from build123d import *
from build123d.topology import SkipClean

# Parameters (mm, degrees)
BOSS_EXTRUDE1_DEPTH  = 20
SKETCH2_W            = 53
SKETCH2_H            = 20
CUT_EXTRUDE1_DEPTH   = 20
FILLET1_R            = 9.75
FILLET1_OF_MIRROR4_R = 9.75
SKETCH4_R            = 2.1
CUT_EXTRUDE3_DEPTH   = 20
FILLET2_R            = 20


with BuildPart() as part:
    # Sketch1 → Boss-Extrude1 (new body)
    with BuildSketch(Plane(origin=(0, 0, 0), x_dir=(1, 0, 0), z_dir=(0, 1, 0))):
        with BuildLine():
            Line((34.641016151, 20), (90, 20))
            Line((90, 20), (90, -20))
            Line((90, -20), (34.641016151, -20))
            Line((34.641016151, -20), (34.641016151, -60))
            Line((34.641016151, -60), (0, -60))
            Line((0, -60), (0, -20))
            Line((0, -20), (0, 20))
            Line((0, 20), (0, 40))
            ThreePointArc((0, 40), (20, 34.641016151), (34.641016151, 20))
        make_face()
    boss_extrude1 = extrude(amount=BOSS_EXTRUDE1_DEPTH)

    # Sketch2 → Cut-Extrude1 (cut)
    with BuildSketch(Plane(origin=(0, 20, 0), x_dir=(1, 0, 0), z_dir=(0, 1, 0))):
        with BuildLine():
            Line((0, 16), (0, -16))
            ThreePointArc((0, -16), (16, 0), (0, 16))
        make_face()
        with Locations((63.5, 0)):
            Rectangle(SKETCH2_W, SKETCH2_H)
    cut_extrude1 = extrude(amount=-CUT_EXTRUDE1_DEPTH, mode=Mode.SUBTRACT)

    # Fillet1
    fillet1_edges = [part.edges().sort_by_distance(p)[0] for p in [
        (90, 10, -20),
        (90, 10, 20),
    ]]
    fillet(fillet1_edges, radius=FILLET1_R)

    # Mirror4: Boss-Extrude1, Cut-Extrude1 across plane
    with SkipClean():  # the faces are left unmerged after this step: merging them gives an invalid solid
        add(boss_extrude1.mirror(Plane(origin=(0, 0, 0), x_dir=(0, 0, 1), z_dir=(1, 0, 0))))
        add(cut_extrude1.mirror(Plane(origin=(0, 0, 0), x_dir=(0, 0, 1), z_dir=(1, 0, 0))), mode=Mode.SUBTRACT)
    add(part.part.scale(1), mode=Mode.REPLACE)  # the faces are merged on a copy

    # Fillet1 of Mirror4
    fillet1_of_mirror4_edges = [part.edges().sort_by_distance(p)[0] for p in [
        (-90, 10, -20),
        (-90, 10, 20),
    ]]
    fillet(fillet1_of_mirror4_edges, radius=FILLET1_OF_MIRROR4_R)

    # Sketch4 → Cut-Extrude3 (cut)
    with BuildSketch(Plane(origin=(0, 20, 0), x_dir=(1, 0, 0), z_dir=(0, 1, 0))):
        with Locations(Location((21, 0, 0), (0, 0, 270))):
            Circle(SKETCH4_R)
        with Locations(Location((14.849242405, -14.849242405, 0), (0, 0, 270))):
            Circle(SKETCH4_R)
        with Locations(Location((0, -21, 0), (0, 0, 270))):
            Circle(SKETCH4_R)
        with Locations(Location((-14.849242405, -14.849242405, 0), (0, 0, 270))):
            Circle(SKETCH4_R)
        with Locations(Location((-21, 0, 0), (0, 0, 270))):
            Circle(SKETCH4_R)
        with Locations(Location((-14.849242405, 14.849242405, 0), (0, 0, 270))):
            Circle(SKETCH4_R)
        with Locations(Location((0, 21, 0), (0, 0, 270))):
            Circle(SKETCH4_R)
        with Locations(Location((14.849242405, 14.849242405, 0), (0, 0, 270))):
            Circle(SKETCH4_R)
    extrude(amount=-CUT_EXTRUDE3_DEPTH, mode=Mode.SUBTRACT)

    # Fillet2
    fillet2_edges = [part.edges().sort_by_distance(p)[0] for p in [
        (34.641016151, 10, 60),
        (-34.641016151, 10, 60),
    ]]
    fillet(fillet2_edges, radius=FILLET2_R)


solid = part.part
Could you check a few things on this model? Use its own coordinates, in mm. A direction names the side the tool comes from. Coordinates: 2 decimals unless noted, no trailing zeros. Order: outer loops, then holes, each group sorted by start corner. A loop starts at its lowest first (then second) coordinate and runs counter-clockwise, first axis right, second up. Notation, with made-up numbers: (41.5, -27) -> (94.5, -27) arc R23 ccw to (94.5, -13) -> close; hole circle Ø4 at (-7, -34). An arc over 180 degrees is marked (long way). One line per question, with ' | ' between items.
Q1. Thinking about a two-plate mould opening in X: for faces 4 (the face through (34.641, 10, 30)), 5 (the face through (58, 10, 20)), 6 (the face through (16.93, 10.14, 14.58)), 7 (the face through (-87.07, 10.14, 17.22)), which applies, pulls with the +X half, pulls with the -X half, needs draft (parallel to the pull), parting line crosses it, or undercut?
Return value:
face 4: pulls with the +X half | face 5: needs draft | face 6: undercut | face 7: pulls with the -X half
Q2. Imagine slicing it at C-C on y = 8. State how many separate pieces and enclosed holes the cut face has, and give its area (3 significant figures).
Return value:
separate pieces: 1 | enclosed holes: 9 | area: 7,670 mm²
Q3. On a 3-axis mill with a long thin cutter (end or side, diameter ignored), from which of +Z, -Z, +X, -X, +Y, -Y can I reach the whole of each face in a straight line? I mean faces 1 (the face through (-12.767, 10.14, 14.576)), 2 (the face through (-63, 10, 10)), 3 (the face through (-58, 10, 20)). Say none if no direction works.
Return value:
face 1: +Y, -Y | face 2: -X, +Y, -Y | face 3: +Z, -X, +Y, -Y
Q4. If I drill on L1, parallel to X at y = 8.25, z = 0; L2, parallel to X at y = 5, z = 21; L3, parallel to Z at x = 57, y = 11, over which ranges is the centre line in solid material (lowest first)?
Return value:
L1: -37 to -23.1, -18.9 to -16, 16 to 18.9, 23.1 to 37 | L2: -34.64 to -2.1, 2.1 to 34.64 | L3: -20 to -10, 10 to 20
Q5. Imagine slicing it at B-B on x = -44. Please give me the cut outline in (y, z), and give its area (3 significant figures).
Return value:
outline: (0, -20) -> (20, -20) -> (20, -10) -> (0, -10) -> close; (0, 10) -> (20, 10) -> (20, 20) -> (0, 20) -> close | area: 400 mm²
Q6. Imagine slicing it at A-A on z = 0. Please give me the cut outline in (x, y).
Return value:
outline: (-37, 0) -> (-23.1, 0) -> (-23.1, 20) -> (-37, 20) -> close; (-18.9, 0) -> (-16, 0) -> (-16, 20) -> (-18.9, 20) -> close; (16, 0) -> (18.9, 0) -> (18.9, 20) -> (16, 20) -> close; (23.1, 0) -> (37, 0) -> (37, 20) -> (23.1, 20) -> close
Q7. Imagine slicing it at D-D on x = 21. Please give me the cut outline in (y, z), and give its area (3 significant figures).
Return value:
outline: (0, -34.04) -> (20, -34.04) -> (20, -2.1) -> (0, -2.1) -> close; (0, 2.1) -> (20, 2.1) -> (20, 58.96) -> (0, 58.96) -> close | area: 1,780 mm²
Q8. I'm going to push flat-ended pins straight in: P1, Ø3.5, axis at x = -14.85, z = 14.85, coming from the -Y side; P2, Ø1.5, axis at x = 5.5, y = 11.5, coming from the -Z side; P3, Ø10, axis at y = 9, z = 26, coming from the +X side; P4, Ø6, axis at x = -61, y = 6.5, coming from the +Z side. Where does each tip first touch, or does it pass through?
Return value:
P1: through | P2: z = -39.72 | P3: x = 34.64 | P4: z = 20
